from build123d import *

# Parameters (mm, degrees)
F1_R     = 33.669764
F3_DEPTH = 25
F0_W     = 33.238638
F0_H     = 92.045456
F4_DEPTH = 25
F2_W     = 54.204546
F2_H     = 28.124999
F5_DEPTH = 25


with BuildPart() as f3:
    # F1 (on Top) → F3 (new body)
    with BuildSketch(Plane.XY):
        with Locations((0, 23.139205)):
            Circle(F1_R)
    extrude(amount=F3_DEPTH)

    # F0 (on Top) → F4 (join)
    with BuildSketch(Plane.XY):
        Rectangle(F0_W, F0_H)
    extrude(amount=F4_DEPTH)

    # F2 (on Top) → F5 (join)
    with BuildSketch(Plane.XY):
        with Locations((0, -38.863636)):
            Rectangle(F2_W, F2_H)
    extrude(amount=F5_DEPTH)


solid = f3.part
Can you work these out from the model? Positions are in its coordinate system, mm. A direction names the side the tool comes from. Give positions to 0.01 mm unless a question says otherwise; leave off trailing zeros. Loops run counter-clockwise (first coordinate to the right, second up) from the corner with the lowest first, then second, coordinate; pieces in that order, holes last. Notation, with made-up numbers: (44.25, 44) -> (69.25, 44) arc R21 cw to (69.25, 65) -> close; hole circle Ø2 at (60.25, 30.5). An arc over 180 degrees is marked (long way). Write item = value, one per line.
1) Suppose I cut it at C-C on y = -11.5. Write out the boundary of the cut face in (x, z).
Check result:
outline = (-16.62, 0) -> (16.62, 0) -> (16.62, 25) -> (-16.62, 25) -> close
2) Suppose I cut it at B-B on x = -19.5. Write out the boundary of the cut face in (y, z), then the cut area to 3 significant figures.
Check result:
outline = (-52.93, 0) -> (-24.8, 0) -> (-24.8, 25) -> (-52.93, 25) -> close; (-4.31, 0) -> (50.59, 0) -> (50.59, 25) -> (-4.31, 25) -> close
area = 2,080 mm2
3) Will these pins go through, and if not, where does the flat tip stop? pin 1 (4 mm diameter, centred on x = 19, y = 36, fed in from -Z); pin 2 (12 mm diameter, centred on y = 43, z = 22, fed in from -X); pin 3 (1 mm diameter, centred on y = 6.5, z = 14.5, fed in from -X); pin 4 (8.5 mm diameter, centred on x = -19.5, z = 14, fed in from +Y).
Check result:
pin_1 = 0
pin_2 = -30.68
pin_3 = -29.55
pin_4 = 53.16
4) I need wall thicknesses on L1, parallel to X at y = -8, z = 2.75; L2, parallel to Y at x = 21, z = 12.5; L3, parallel to X at y = -26.5, z = 1.75. Which ranges of each line are inside material? Lowest first, please. Write a range as from..to.
Check result:
L1 = -16.62..16.62
L2 = -52.93..-24.8, -3.18..49.46
L3 = -27.1..27.1
5) Suppose I cut it at D-D on y = 38. Write out the boundary of the cut face in (x, z).
Check result:
outline = (-30.21, 0) -> (30.21, 0) -> (30.21, 25) -> (-30.21, 25) -> close
6) Suppose I cut it at A-A on z = 21.25. Write out the boundary of the cut face in (x, y).
Check result:
outline = (-27.1, -52.93) -> (27.1, -52.93) -> (27.1, -24.8) -> (16.62, -24.8) -> (16.62, -6.14) arc R33.67 ccw (long way) to (-16.62, -6.14) -> (-16.62, -24.8) -> (-27.1, -24.8) -> close
7) Thinking about a two-plate mould opening in Y: for faces 4 (the cylindrical face through (1.237, 56.786, 12.325)), 5 (the flat face through (0, 3, 25)), 6 (the flat face through (0, -52.926, 12)), which applies, released by +Y, released by -Y, zero draft, split by the parting line, or undercut?
Check result:
face_4 = undercut
face_5 = zero draft
face_6 = released by -Y
8) For faces 1 (the flat face through (-22, -24.801, 12)), 2 (the flat face through (-27.102, -39, 12)), 3 (the flat face through (22, -24.801, 12)), which set-ups out of +Z, -Z, +X, -X, +Y, -Y let a thin tool reach every point of the face, with its end or its side?
Check result:
face_1 = +Z, -Z, -X
face_2 = +Z, -Z, -X, -Y
face_3 = +Z, -Z, +X
